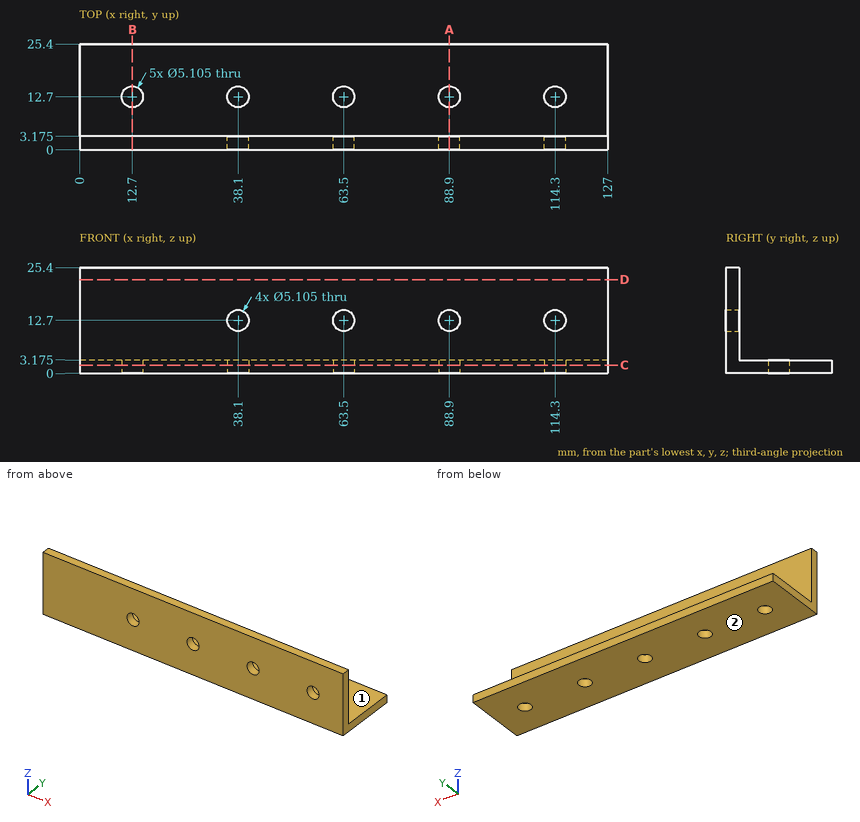
Geometry: see drawing. Coordinates: mm, zero at the bounding-box minimum. A direction names the side the tool comes from. Round coordinates to 2 decimals unless told otherwise and drop trailing zeros. Write each loop counter-clockwise with the first axis right and the second up, starting at its lowest first coordinate (ties: lowest second). Pieces come first, ordered by that corner, then holes. Notation, with made-up numbers: M 36.25,-18 L 55.25,-18 A19 cw 55.25,-10 Z; hole C 30.5,-32.5 d6. An arc over 180 degrees is marked long. Answer in a Markdown table with one row per item. Add a question column.
(1) Ray query, L1, parallel to Z at x = 114.3, y = 1; L2, parallel to Y at x = 68, z = 3.75 (1 decimal). Return the intervals inside material, ascending.
(2) Cut plane A-A, the plane x = 88.9. Return the cut outline in (y, z) (1 decimal), then the cut area to 3 significant figures.
(3) Cut plane C-C, the plane z = 2. Return the cut outline in (x, y) (1 decimal), then the cut area to 3 significant figures.
(4) Cut plane B-B, the plane x = 12.7. Return the cut outline in (y, z) (1 decimal), then the cut area to 3 significant figures.
(5) Reachability of the marked faces 1 and 2 from +Z, -Z, +X, -X, +Y, -Y: full face, straight path, thin tool, end or side. Return the list, or none.
(6) Cut plane D-D, the plane z = 22.5. Return the cut outline in (x, y) (1 decimal), then the cut area to 3 significant figures.
(7) Contact query for flat-ended pins moving along their axis: pin 1 (8 mm diameter, centred on x = 81, z = 17.5, fed in from +Y) (3 decimals); pin 2 (8 mm diameter, centred on x = 63.5, y = 12.7, fed in from +Z) (3 decimals). Output: stop coordinate, or through.
Established:
| question | item | result |
|---|---|---|
| 1 | L1 | 0 to 10.15, 15.25 to 25.4 |
| 1 | L2 | 0 to 3.2 |
| 2 | outline | M 0,0 L 10.1,0 L 10.1,3.2 L 3.2,3.2 L 3.2,10.1 L 0,10.1 Z; M 0,15.3 L 3.2,15.3 L 3.2,25.4 L 0,25.4 Z; M 15.3,0 L 25.4,0 L 25.4,3.2 L 15.3,3.2 Z |
| 2 | area | 119 mm² |
| 3 | outline | M 0,0 L 127,0 L 127,25.4 L 0,25.4 Z; hole C 12.7,12.7 d5.1; hole C 38.1,12.7 d5.1; hole C 63.5,12.7 d5.1; hole C 88.9,12.7 d5.1; hole C 114.3,12.7 d5.1 |
| 3 | area | 3,120 mm² |
| 4 | outline | M 0,0 L 10.1,0 L 10.1,3.2 L 3.2,3.2 L 3.2,25.4 L 0,25.4 Z; M 15.3,0 L 25.4,0 L 25.4,3.2 L 15.3,3.2 Z |
| 4 | area | 135 mm² |
| 5 | face 1 | +Z, +X, -X, +Y |
| 5 | face 2 | -Z, +X, -X, +Y, -Y |
| 6 | outline | M 0,0 L 127,0 L 127,3.2 L 0,3.2 Z |
| 6 | area | 403 mm² |
| 7 | pin 1 | y = 3.175 |
| 7 | pin 2 | z = 3.175 |
